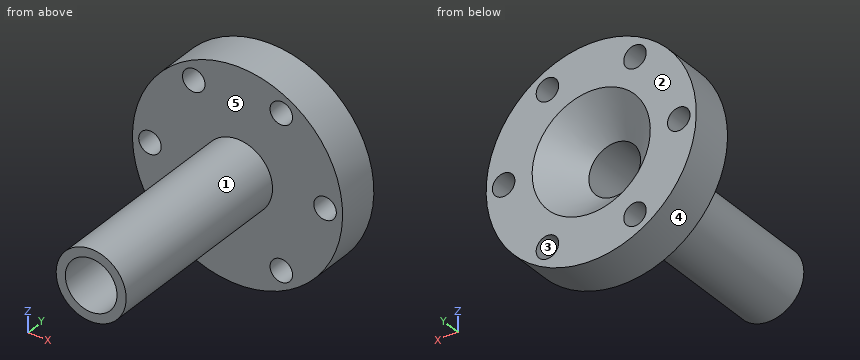
```python
from build123d import *

# Parameters (mm, degrees)
F_1_4_CLEARANCE_HOLE1_D = 6.5278
CIRPATTERN1_COUNT       = 6


with BuildPart() as part:
    # Sketch1 → Revolve1 (revolve)
    with BuildSketch(Plane.XY, mode=Mode.PRIVATE) as revolve1_sk:
        Polygon((7.5, -72.82), (7.5, -9.645), (17.145, 0), (30.48, 0), (30.48, -12.82), (10.16, -12.82), (10.16, -72.82), align=None)
    revolve(revolve1_sk.sketch.rotate(Axis((0, 0, 0), (0, -1, 0)), 90), axis=Axis((0, 0, 0), (0, -1, 0)))

    # 1/4 Clearance Hole1 (through all)
    with Locations(Plane(origin=(0, 0, 0), x_dir=(1, 0, 0), z_dir=(0, 1, 0))):
        with Locations((25.4, 0)):
            f_1_4_clearance_hole1 = Hole(F_1_4_CLEARANCE_HOLE1_D / 2)

    # CirPattern1: 1/4 Clearance Hole1 ×6 about axis
    cirpattern1_axis = Axis((0, 0, 0), (0, 1, 0))
    for i in range(1, CIRPATTERN1_COUNT):
        add(f_1_4_clearance_hole1.rotate(cirpattern1_axis, i * 360 / CIRPATTERN1_COUNT), mode=Mode.SUBTRACT)


solid = part.part
```
CAD build for the part. Positions are in the model's coordinates, mm. Face numbers are marked on the shaded views. A direction names the side the tool comes from. Round coordinates to 2 decimals unless told otherwise and drop trailing zeros. Order: outer loops, then holes, each group sorted by start corner. A loop starts at its lowest first (then second) coordinate and runs counter-clockwise, first axis right, second up.
Q1. Two-plate mould, pull along X, no slides. Class the marked faces 1, 2 and 3: pulls with the +X half, pulls with the -X half, needs draft (parallel to the pull), parting line crosses it, or undercut.
Q2. Slice it at D-D (x = -27). Write the cut outline in (y, z), and give its area (3 significant figures).
Q3. Drop flat-ended pins along their axis: pin 1 (10 mm diameter, centred on x = 5, z = -21.5, fed in from -Y); pin 2 (5 mm diameter, centred on y = -56, z = 5.5, fed in from +X); pin 3 (10 mm diameter, centred on x = 3.5, y = -44.5, fed in from -Z). Give the stop position or say it passes through.
Q4. Slice it at A-A (z = 0). Write the cut outline in (x, y) (3 decimals).
Q5. Wall check: L1, parallel to X at y = -48, z = 0; L2, parallel to Y at x = 24.5, z = 13.5; L3, parallel to Z at x = 12.7, y = -9.75. Give the ranges that are in metal, low to high.
Q6. Slice it at C-C (y = -41.5). Write the cut outline in (x, z), and give its area (3 significant figures).
Q7. Which spindle directions (+Z, -Z, +X, -X, +Y, -Y) get a long thin tool onto all of the face, cutting with end or side? Do the marked faces 4 and 5. Say none if no direction does.
Q8. Slice it at B-B (x = 25.4). Write the cut outline in (y, z).
Results below:
1. face 1: parting line crosses it
1. face 2: needs draft
1. face 3: undercut
2. outline: (-12.82, -14.14) - (0, -14.14) - (0, -2.84) - (-12.82, -2.84) - close; (-12.82, 2.84) - (0, 2.84) - (0, 14.14) - (-12.82, 14.14) - close
2. area: 290 mm2
3. pin 1: stops at y = -12.82
3. pin 2: stops at x = 9.71
3. pin 3: stops at z = -10.16
4. outline: (-30.48, -12.82) - (-28.664, -12.82) - (-28.664, 0) - (-30.48, 0) - close; (-22.136, -12.82) - (-10.16, -12.82) - (-10.16, -72.82) - (-7.5, -72.82) - (-7.5, -9.645) - (-17.145, 0) - (-22.136, 0) - close; (7.5, -72.82) - (10.16, -72.82) - (10.16, -12.82) - (22.136, -12.82) - (22.136, 0) - (17.145, 0) - (7.5, -9.645) - close; (28.664, -12.82) - (30.48, -12.82) - (30.48, 0) - (28.664, 0) - close
5. L1: x = -10.16 to -7.5, 7.5 to 10.16
5. L2: y = -12.82 to 0
5. L3: z = -27.71 to -25.26, -18.73 to 18.73, 25.26 to 27.71
6. outline: circle Ø20.32 at (0, 0); hole circle Ø15 at (0, 0)
6. area: 148 mm2
7. face 4: +Y, -Y
7. face 5: -Y
8. outline: (-12.82, -16.85) - (0, -16.85) - (0, -3.26) - (-12.82, -3.26) - close; (-12.82, 3.26) - (0, 3.26) - (0, 16.85) - (-12.82, 16.85) - close
